```python
from build123d import *

# Parameters (mm, degrees)
F1_DEPTH = 5
F2_SIZE  = 4.99999


# Not quite as in the source:
# - a fillet or chamfer is up to 0.001 mm smaller than in the source, because OpenCascade refuses the exact size


with BuildPart() as f1:
    # F0 (on Top) → F1 (new body)
    with BuildSketch(Plane.XY):
        Polygon((-27.5, -11.5), (27.5, -14.74), (27.5, 52.5), (-27.5, 52.5), align=None)
        Polygon((-27.5, -14.74), (27.5, -14.74), (-27.5, -11.5), align=None)
    extrude(amount=F1_DEPTH)

    # F2 (size 5 in the source; OpenCascade refuses exactly that, so slightly less here)
    f2_edges = [f1.edges().sort_by_distance(p)[0] for p in [
        (27.5, 18.88, 0),
        (0, 52.5, 0),
        (-27.5, 18.88, 0),
    ]]
    chamfer(f2_edges, length=F2_SIZE)


solid = f1.part
```
Work out the finished part from the listing and answer in its coordinate system (mm). Give positions to 0.01 mm unless a question says otherwise; leave off trailing zeros. Loops run counter-clockwise (first coordinate to the right, second up) from the corner with the lowest first, then second, coordinate; pieces in that order, holes last. Notation, with made-up numbers: (6.5, -33) -> (32.5, -33) arc R36 ccw to (32.5, 4) -> close; hole circle Ø6 at (16.25, -12.75). An arc over 180 degrees is marked (long way). Write item = value, one per line. Start each with the question number.
(1) Find the intervals of material crossed by probe 1 along Y at (x, z) = (8, 0.8); probe 2 along Y at (x, z) = (-22, 4.4); probe 3 along X at (y, z) = (-3.5, 4.2), in increasing order. Write a range as from..to.
(2) Find section C-C on z = 1.85. Give the vertices of the cut face in (x, y).
(3) Given pin 1 Ø1 at (y, z) = (0, 3) entering from +X; pin 2 Ø3 at (y, z) = (6, 4) entering from +X, each flat-ended and moving along its own axis, determine where each tip first touches the part or whether it passes through.
From the geometry:
q1.probe_1 = -14.74..48.3
q1.probe_2 = -14.74..51.9
q1.probe_3 = -26.7..26.7
q2.outline = (-24.35, -14.74) -> (24.35, -14.74) -> (24.35, 49.35) -> (-24.35, 49.35) -> close
q3.pin_1 = 26
q3.pin_2 = 27.5
